from build123d import *

# Parameters (mm, degrees)
F0_W      = 52
F0_H      = 15
F1_DEPTH  = 45
F2_DEPTH  = 61
F4_DEPTH  = 15
F6_R      = 9
F5_R      = 9
F7_DEPTH  = 15
F10_DEPTH = 30


with BuildPart() as f1:
    # F0 (on Front) → F1 (new body)
    with BuildSketch(Plane.XZ):
        with Locations((-56.5, -23)):
            Rectangle(F0_W, F0_H)
    extrude(amount=F1_DEPTH)



with BuildPart() as f1b:
    # F0 (on Front) → F1, piece 2 (new body)
    with BuildSketch(Plane.XZ):
        with Locations((56.5, -23)):
            Rectangle(F0_W, F0_H)
    extrude(amount=F1_DEPTH)


with BuildPart() as f1_1:
    add(f1.part)

    add(f1b.part)  # F2 merges F1b
    # F0 (on Front) → F2 (join)
    with BuildSketch(Plane.XZ):
        Polygon((30.5, 30.5), (-30.5, 30.5), (-30.5, -15.5), (-30.5, -30.5), (30.5, -30.5), (30.5, -15.5), align=None)
    extrude(amount=F2_DEPTH)

    # F3 (on face) → F4 (join)
    with BuildSketch(Plane.XY.offset(-15.5)):
        with BuildLine():
            Line((-82.5, -45), (-82.5, 0))
            ThreePointArc((-82.5, 0), (-105, -22.5), (-82.5, -45))
        make_face()
        with BuildLine():
            Line((82.5, 0), (82.5, -45))
            ThreePointArc((82.5, -45), (105, -22.5), (82.5, 0))
        make_face()
    extrude(amount=-F4_DEPTH)

    # F6 (on face) + F5 (on face) → F7 (cut)
    with BuildSketch(Plane.XY.offset(-15.5)):
        with Locations((82.5, -22.5)):
            Circle(F6_R)
    with BuildSketch(Plane.XY.offset(-15.5)):
        with Locations((-82.5, -22.5)):
            Circle(F5_R)
    extrude(amount=-F7_DEPTH, mode=Mode.SUBTRACT)

    # F9 (on offset) → F10 (cut)
    with BuildSketch(Plane(origin=(-15, 0, 0), x_dir=(0, -1, 0), z_dir=(-1, 0, 0))):
        Polygon((61, 30.5), (13.75, 30.5), (53, -30.5), (61, -30.5), align=None)
    extrude(amount=-F10_DEPTH, mode=Mode.SUBTRACT)


solid = f1_1.part
Design review of the part built by this model. Coordinates are the model's own, in mm. A direction names the side the tool comes from. Coordinates: 2 decimals unless noted, no trailing zeros. Loops run counter-clockwise (first coordinate to the right, second up) from the corner with the lowest first, then second, coordinate; pieces in that order, holes last.
Item 1: Clearance check with flat-ended pins moving along their axes: pin 1 (1 mm diameter, centred on y = -42.5, z = 12.5, fed in from -X); pin 2 (10 mm diameter, centred on y = -48, z = -5, fed in from +X); pin 3 (22.5 mm diameter, centred on x = -85.5, y = -23, fed in from +Z); pin 4 (23.5 mm diameter, centred on x = -82.5, y = -22.5, fed in from -Z). State where each tip first meets the part, or that it passes through.
Completed:
pin 1: stops at x = -30.5
pin 2: stops at x = 30.5
pin 3: stops at z = -15.5
pin 4: stops at z = -30.5
Item 2: Add section C-C (y = -4). Write out the cut boundary in (x, z).
Completed:
outline: (-95.31, -30.5) - (95.31, -30.5) - (95.31, -15.5) - (30.5, -15.5) - (30.5, 30.5) - (-30.5, 30.5) - (-30.5, -15.5) - (-95.31, -15.5) - close
Item 3: Add section B-B (z = -22). Write out the cut boundary in (x, y).
Completed:
outline: (-82.5, -45) - (-30.5, -45) - (-30.5, -61) - (-15, -61) - (-15, -47.53) - (15, -47.53) - (15, -61) - (30.5, -61) - (30.5, -45) - (82.5, -45) arc R22.5 ccw to (82.5, 0) - (-82.5, 0) arc R22.5 ccw to start; hole circle Ø18 at (-82.5, -22.5); hole circle Ø18 at (82.5, -22.5)
Item 4: Add section A-A (x = -78). Write out the cut boundary in (y, z), and give its area (3 significant figures).
Completed:
outline: (-45, -30.5) - (-30.29, -30.5) - (-30.29, -15.5) - (-45, -15.5) - close; (-14.71, -30.5) - (0, -30.5) - (0, -15.5) - (-14.71, -15.5) - close
area: 441 mm2
Item 5: Draft analysis for pull direction Y (two halves, no side actions). For faces 4 (the flat face through (67, -22, -15.5)), 5 (the flat face through (-1, 0, -6)), 6 (the cylindrical face through (91.084, -19.797, -22.895)), state which applies: pulls with the +Y half, pulls with the -Y half, needs draft (parallel to the pull), parting line crosses it, or undercut.
Completed:
face 4: needs draft
face 5: pulls with the +Y half
face 6: undercut
Item 6: For faces 1 (the flat face through (-68, -22, -15.5)), 2 (the flat face through (56, -45, -23)), 3 (the flat face through (-15, -42, 7)), list the 3-axis set-ups (+Z, -Z, +X, -X, +Y, -Y) from which the entire face can be reached by the end or side of a thin tool; tool diameter is ignored.
Completed:
face 1: +Z, -X, +Y, -Y
face 2: +Z, -Z, +X, -Y
face 3: +Z, -Y
Item 7: Add section D-D (x = 48). Write out the cut boundary in (y, z).
Completed:
outline: (-45, -30.5) - (0, -30.5) - (0, -15.5) - (-45, -15.5) - close
Item 8: Wall thickness on L1, parallel to X at y = -22, z = -20; L2, parallel to Y at x = 82, z = -23; L3, parallel to Z at x = -73, y = -27.5: over which ranges is each line inside the solid? List them lowest first.
Completed:
L1: x = -104.99 to -91.49, -73.51 to 73.51, 91.49 to 104.99
L2: y = -45 to -31.49, -13.51 to 0
L3: z = -30.5 to -15.5
